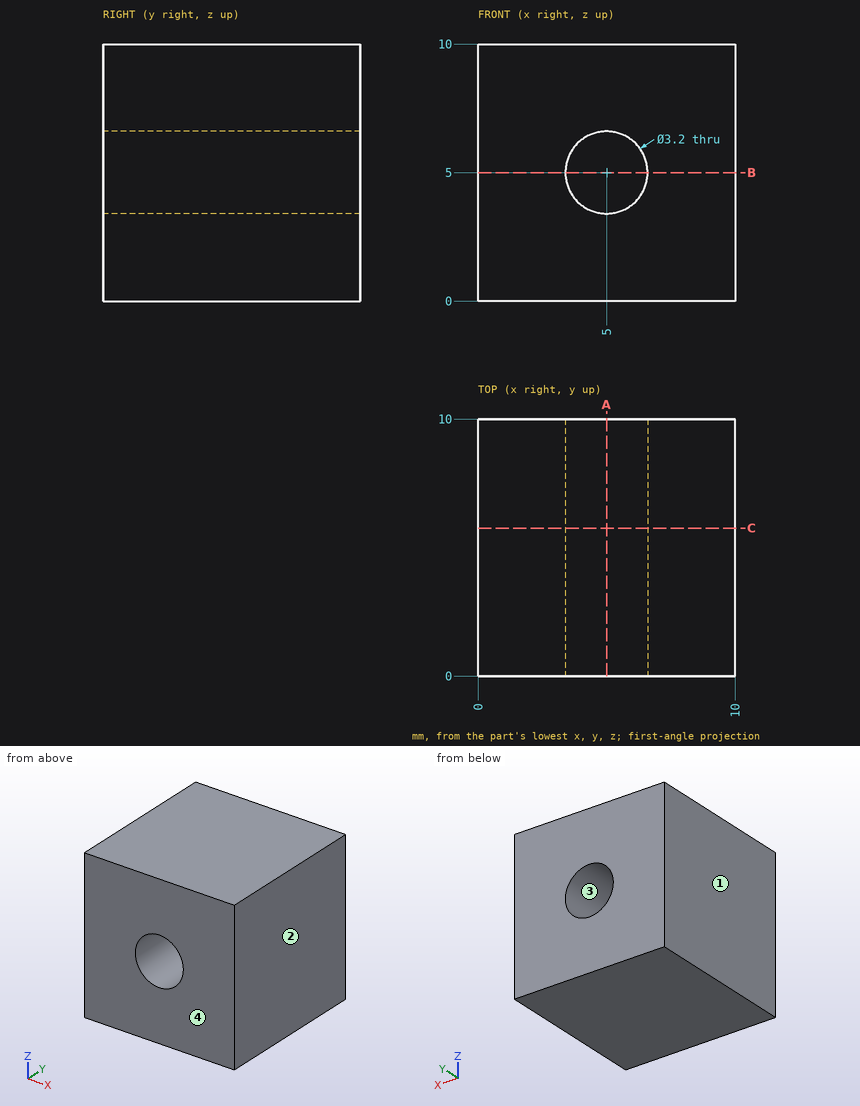
Job drawing, mm, ordinate dimensions from the low corner. One solid piece. Coordinates: 2 decimals unless noted, no trailing zeros. Write each loop counter-clockwise with the first axis right and the second up, starting at its lowest first coordinate (ties: lowest second). Pieces come first, ordered by that corner, then holes. Notation, with made-up numbers: M 76.5,79 L 127.5,79 A25 cw 127.5,99 Z; hole C -28,-21.5 d1. An arc over 180 degrees is marked long. Answer as a JSON object with one key per item and string values. Group by question number.
1) Mould opens along X. For the marked faces 1, 2, 3 and 4 say: +X half, -X half, draft (parallel to the pull), parting line (faces both ways), or undercut.
2) Saw through at B-B (z = 5). Write the cut outline in (x, y), plus the area to 3 significant figures.
3) Saw through at C-C (y = 5.75). Write the cut outline in (x, z), plus the area to 3 significant figures.
4) Wall check: line 1 (X direction, y = 6.5, z = 5); line 2 (X direction, y = 9.75, z = 4.5). Give the ranges that are in metal, low to high. Write a range as from..to.
5) Saw through at A-A (x = 5). Write the cut outline in (y, z).
Values follow:
{
 "1": {"face 1": "-X half", "face 2": "+X half", "face 3": "undercut", "face 4": "draft"},
 "2": {"outline": "M 0,0 L 3.4,0 L 3.4,10 L 0,10 Z; M 6.6,0 L 10,0 L 10,10 L 6.6,10 Z", "area": "68.0 mm2"},
 "3": {"outline": "M 0,0 L 10,0 L 10,10 L 0,10 Z; hole C 5,5 d3.2", "area": "92.0 mm2"},
 "4": {"line 1": "x = 0..3.4, 6.6..10", "line 2": "x = 0..3.48, 6.52..10"},
 "5": {"outline": "M 0,0 L 10,0 L 10,3.4 L 0,3.4 Z; M 0,6.6 L 10,6.6 L 10,10 L 0,10 Z"}
}
